from build123d import *

# Parameters (mm, degrees)
F0_R     = 9.053492
F0_R_2   = 8.043979
F1_DEPTH = 25.4
F2_W     = 16.844214
F2_H     = 62.323578
F3_DEPTH = 45.974
F5_DEPTH = 25.4
F6_R     = 4.361734
F7_DEPTH = 85.598


with BuildPart() as f1:
    # F0 (on Top) → F1 (new body)
    with BuildSketch(Plane.XY):
        with BuildLine():
            Line((14.598317, -57.270318), (14.598317, 57.270318))
            ThreePointArc((14.598317, 57.270318), (0, 71.868635), (-14.598317, 57.270318))
            Line((-14.598317, 57.270318), (-14.598317, -57.270318))
            ThreePointArc((-14.598317, -57.270318), (0, -71.868635), (14.598317, -57.270318))
        make_face()
        with Locations((0, -57.270318)):
            Circle(F0_R, mode=Mode.SUBTRACT)
        with Locations((0, 57.270318)):
            Circle(F0_R_2, mode=Mode.SUBTRACT)
    extrude(amount=F1_DEPTH)

    # F2 (on face) → F3 (join)
    with BuildSketch(Plane.XY.offset(25.4)):
        Rectangle(F2_W, F2_H)
    extrude(amount=F3_DEPTH)

    # F4 (on face) → F5 (cut)
    with BuildSketch(Plane.YZ.offset(8.422107)):
        with BuildLine():
            Line((7.322163, 71.374), (-9.203623, 71.374))
            Line((-9.203623, 71.374), (-9.203623, 38.925104))
            ThreePointArc((-9.203623, 38.925104), (-1.024193, 30.578748), (7.322163, 38.758177))
            Line((7.322163, 38.758177), (7.322163, 71.374))
        make_face()
    extrude(amount=-F5_DEPTH, mode=Mode.SUBTRACT)

    # F6 (on face) → F7 (cut)
    with BuildSketch(Plane.XZ.offset(31.161789)):
        with BuildLine():
            Line((-8.422107, 71.374), (-8.422107, 59.979465))
            ThreePointArc((-8.422107, 59.979465), (0, 68.401572), (8.422107, 59.979465))
            Line((8.422107, 59.979465), (8.422107, 71.374))
            Line((8.422107, 71.374), (-8.422107, 71.374))
        make_face()
        with Locations((0, 59.979465)):
            Circle(F6_R)
    extrude(amount=-F7_DEPTH, mode=Mode.SUBTRACT)


solid = f1.part
For this review, take the finished solid that the model builds, in its own axes (mm). A direction names the side the tool comes from. Round coordinates to 2 decimals unless told otherwise and drop trailing zeros. Write each loop counter-clockwise with the first axis right and the second up, starting at its lowest first coordinate (ties: lowest second). Pieces come first, ordered by that corner, then holes. Notation, with made-up numbers: M 64.5,36.25 L 112.5,36.25 A16 cw 112.5,48.25 Z; hole C -8,79 d9. An arc over 180 degrees is marked long. Write item = value, one per line. Start each with the question number.
(1) For line 1 along Y through (x, z) = (0, 15.25); line 2 along Y through (x, z) = (-6, 58); line 3 along Z through (x, y) = (0, 12.5), list the stretches that pass through material, from the lowest coordinate up.
(2) For faces 1 (the face through (0, 31.162, 47)), 2 (the face through (8.422, 6.5, 34.8)), 3 (the face through (0, -9.204, 51)), 4 (the face through (-8.422, 6.5, 34.8)), 5 (the face through (0, -31.162, 47)), list the 3-axis set-ups (+Z, -Z, +X, -X, +Y, -Y) from which the entire face can be reached by the end or side of a thin tool; tool diameter is ignored.
(3) Clearance check with flat-ended pins moving along their axes: pin 1 Ø5 at (y, z) = (-23.5, 56.5) entering from +X; pin 2 Ø1 at (x, z) = (5.5, 24) entering from -Y; pin 3 Ø13.5 at (x, z) = (0.5, 37) entering from -Y. State where each tip first meets the part, or that it passes through.
(4) The part is to be moulded in two halves that separate along X. For faces 6 (the face through (-0.6, 19.1, 64.3)), 7 (the face through (-0.321, -71.865, 12.522)), 8 (the face through (0.118, -1.206, 30.583)), 9 (the face through (3.712, 50.134, 12.522)), say which applies: +X half, -X half, draft (parallel to the pull), parting line (faces both ways), or undercut.
(5) We need section A-A (z = 42). Give the boundary of the cut face in (x, y).
(6) We need section D-D (z = 12.5). Give the boundary of the cut face in (x, y), then the cut area to 3 significant figures.
(7) We need section C-C (y = -22). Give the boundary of the cut face in (x, z), then the cut area to 3 significant figures.
(8) We need section B-B (x = 0). Give the boundary of the cut face in (y, z).
Results found:
q1.line_1 = -71.87 to -66.32, -48.22 to 49.23, 65.31 to 71.87
q1.line_2 = -31.16 to -9.2, 7.32 to 31.16
q1.line_3 = 0 to 55.62, 64.34 to 68.4
q2.face_1 = +Z, +X, -X, +Y
q2.face_2 = +Z, +X, +Y, -Y
q2.face_3 = +Z, +X, -X
q2.face_4 = +Z, -X, +Y, -Y
q2.face_5 = +Z, +X, -X, -Y
q3.pin_1 = 8.42
q3.pin_2 = -70.99
q3.pin_3 = -31.16
q4.face_6 = undercut
q4.face_7 = parting line
q4.face_8 = draft
q4.face_9 = undercut
q5.outline = M -8.42,-31.16 L 8.42,-31.16 L 8.42,-9.2 L -8.42,-9.2 Z; M -8.42,7.32 L 8.42,7.32 L 8.42,31.16 L -8.42,31.16 Z
q6.outline = M -14.6,-57.27 A14.6 ccw 14.6,-57.27 L 14.6,57.27 A14.6 ccw -14.6,57.27 Z; hole C 0,-57.27 d18.11; hole C 0,57.27 d16.09
q6.area = 3,550 mm²
q7.outline = M -14.6,0 L 14.6,0 L 14.6,25.4 L 8.42,25.4 L 8.42,59.98 A8.42 ccw -8.42,59.98 L -8.42,25.4 L -14.6,25.4 Z; hole C 0,59.98 d8.72
q7.area = 1,380 mm²
q8.outline = M -71.87,0 L -66.32,0 L -66.32,25.4 L -71.87,25.4 Z; M -48.22,0 L 49.23,0 L 49.23,25.4 L 31.16,25.4 L 31.16,55.62 L 7.32,55.62 L 7.32,38.76 A8.26 cw -9.2,38.93 L -9.2,55.62 L -31.16,55.62 L -31.16,25.4 L -48.22,25.4 Z; M -31.16,64.34 L -9.2,64.34 L -9.2,68.4 L -31.16,68.4 Z; M 7.32,64.34 L 31.16,64.34 L 31.16,68.4 L 7.32,68.4 Z; M 65.31,0 L 71.87,0 L 71.87,25.4 L 65.31,25.4 Z
